Geometry: final body of the model. Coordinates: model frame, mm. Face numbers are marked on the shaded views. Coordinates: 2 decimals unless noted, no trailing zeros. Loops run counter-clockwise (first coordinate to the right, second up) from the corner with the lowest first, then second, coordinate; pieces in that order, holes last. Notation, with made-up numbers: (57, 43.25) - (75, 43.25) arc R15 cw to (75, 69.25) - close; hole circle Ø4 at (22.5, -7.75). An arc over 180 degrees is marked (long way). Answer in a Markdown table with one row per item.
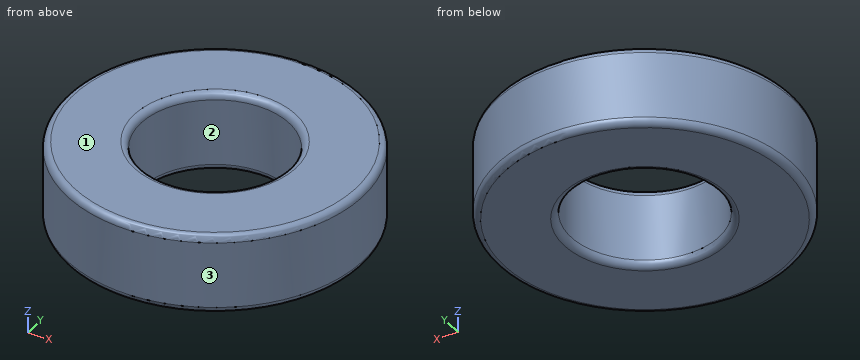
from build123d import *

# Parameters (mm, degrees)
F0_R     = 5.5565
F1_DEPTH = 3
F2_D     = 5.588
F3_R     = 0.25


with BuildPart() as f1:
    # F0 (on Top) → F1 (new body)
    with BuildSketch(Plane.XY):
        Circle(F0_R)
    extrude(amount=F1_DEPTH)

    # F2 (through all)
    with Locations(Plane(origin=(0, 0, 0), x_dir=(1, 0, 0), z_dir=(0, 0, -1))):
        with Locations((0, 0)):
            Hole(F2_D / 2)

    # F3
    f3_edges = [f1.edges().sort_by_distance(p)[0] for p in [
        (-5.5565, 0, 0),
        (-5.5565, 0, 3),
        (-2.794, 0, 3),
        (-2.794, 0, 0),
    ]]
    fillet(f3_edges, radius=F3_R)


solid = f1.part
(1) Cut plane A-A on y = 0. Output: boundary loops of the cut face in (x, z).
Verdict:
| item | result |
|---|---|
| outline | (-5.56, 0.25) arc R0.25 ccw to (-5.31, 0) - (-3.04, 0) arc R0.25 ccw to (-2.79, 0.25) - (-2.79, 2.75) arc R0.25 ccw to (-3.04, 3) - (-5.31, 3) arc R0.25 ccw to (-5.56, 2.75) - close; (2.79, 0.25) arc R0.25 ccw to (3.04, 0) - (5.31, 0) arc R0.25 ccw to (5.56, 0.25) - (5.56, 2.75) arc R0.25 ccw to (5.31, 3) - (3.04, 3) arc R0.25 ccw to (2.79, 2.75) - close |
(2) Ray query, probe 1 along Y at (x, z) = (0, 1.7); probe 2 along Y at (x, z) = (1.75, 1.1); probe 3 along X at (y, z) = (-0.5, 1.85). Return the intervals inside material, ascending.
Verdict:
| item | result |
|---|---|
| probe 1 | y = -5.56 to -2.79, 2.79 to 5.56 |
| probe 2 | y = -5.27 to -2.18, 2.18 to 5.27 |
| probe 3 | x = -5.53 to -2.75, 2.75 to 5.53 |
(3) Cut plane C-C on z = 0.6. Output: boundary loops of the cut face in (x, y), then the cut area to 3 significant figures.
Verdict:
| item | result |
|---|---|
| outline | circle Ø11.11 at (0, 0); hole circle Ø5.59 at (0, 0) |
| area | 72.5 mm² |
(4) Pull-direction query (Y, two-part tool) for the marked faces 1, 2 and 3; classes: pulls with the +Y half, pulls with the -Y half, needs draft (parallel to the pull), parting line crosses it, or undercut.
Verdict:
| item | result |
|---|---|
| face 1 | needs draft |
| face 2 | undercut |
| face 3 | parting line crosses it |
(5) First-contact query: pin 1 Ø1.5 at (y, z) = (1, 2.5) entering from +X. Flat tip, straight axial feed; report the tip coordinate or a pass-through.
Verdict:
| item | result |
|---|---|
| pin 1 | stops at x = 5.55 |
